The listing builds one solid part. Answer for the finished solid, in the listing's coordinates (mm). Coordinates: 2 decimals unless noted, no trailing zeros. Loops run counter-clockwise (first coordinate to the right, second up) from the corner with the lowest first, then second, coordinate; pieces in that order, holes last. Notation, with made-up numbers: M 42.25,55 L 99.25,55 A19 ccw 99.25,65 Z; hole C -18,-19.5 d1. An arc over 180 degrees is marked long. Return JSON: item names as keys, results as strings. Group by question number.
1. Section B-B (y = 124) is taken. Write down the section's boundary in (x, z).
2. Straight lines are drawn through the part: L1, parallel to Y at x = 82.5, z = 3.5; L2, parallel to X at y = 96, z = 3.8; L3, parallel to Y at x = 133, z = 1.1. For each, find the intervals that lie inside material, in ascending order. Write a range as from..to.
3. Section A-A (y = 19.05) is taken. Write down the section's boundary in (x, z) (3 decimals).
4. Given P1, Ø2, axis at x = 85.5, z = 1.5, coming from the +Y side; P2, Ø2, axis at x = 2, z = 2, coming from the +Y side; P3, Ø2, axis at y = 75.5, z = 1.5, coming from the +X side, each flat-ended and moving along its own axis, determine where each tip first touches the part or whether it passes through.
```python
from build123d import *

# Parameters (mm, degrees)
BOSS_EXTRUDE1_DEPTH = 4.4958
FILLET1_R           = 12.7
SKETCH2_W           = 4.4958
SKETCH2_H           = 12.7
CUT_EXTRUDE1_DEPTH  = 302.762747772
SKETCH3_W           = 12.7
SKETCH3_H           = 4.4958
CUT_EXTRUDE2_DEPTH  = 302.762747772
SKETCH4_R           = 5.08
CUT_EXTRUDE3_DEPTH  = 302.762747772
SKETCH5_W           = 25.4
SKETCH5_H           = 6.35
CUT_EXTRUDE4_DEPTH  = 302.762747772


with BuildPart() as part:
    # Sketch1 → Boss-Extrude1 (new body)
    with BuildSketch(Plane.XY):
        with BuildLine():
            Line((0, 114.3), (0, 0))
            Line((0, 0), (248.285, 0))
            Line((248.285, 0), (248.285, 114.3))
            ThreePointArc((248.285, 114.3), (207.873847455, 131.038847455), (191.135, 171.45))
            Line((191.135, 171.45), (57.15, 171.45))
            ThreePointArc((57.15, 171.45), (40.411152545, 131.038847455), (0, 114.3))
        make_face()
    extrude(amount=BOSS_EXTRUDE1_DEPTH)

    # Fillet1
    fillet1_edges = [part.edges().sort_by_distance(p)[0] for p in [
        (248.285, 114.3, 2.2479),
        (0, 114.3, 2.2479),
        (57.15, 171.45, 2.2479),
        (191.135, 171.45, 2.2479),
    ]]
    fillet(fillet1_edges, radius=FILLET1_R)

    # Sketch2 → Cut-Extrude1 (cut, through all)
    with BuildSketch(Plane.XY.offset(4.4958)):
        with Locations((246.0371, 96.414248202)):
            Rectangle(SKETCH2_W, SKETCH2_H)
        with Locations((246.0371, 77.364248202)):
            Rectangle(SKETCH2_W, SKETCH2_H)
        with Locations((246.0371, 39.264248202)):
            Rectangle(SKETCH2_W, SKETCH2_H)
        with Locations((246.0371, 58.314248202)):
            Rectangle(SKETCH2_W, SKETCH2_H)
        with Locations((246.0371, 20.214248202)):
            Rectangle(SKETCH2_W, SKETCH2_H)
        with Locations((2.2479, 96.414248202)):
            Rectangle(SKETCH2_W, SKETCH2_H)
        with Locations((2.2479, 77.364248202)):
            Rectangle(SKETCH2_W, SKETCH2_H)
        with Locations((2.2479, 58.314248202)):
            Rectangle(SKETCH2_W, SKETCH2_H)
        with Locations((2.2479, 39.264248202)):
            Rectangle(SKETCH2_W, SKETCH2_H)
        with Locations((2.2479, 20.214248202)):
            Rectangle(SKETCH2_W, SKETCH2_H)
    extrude(amount=-CUT_EXTRUDE1_DEPTH, mode=Mode.SUBTRACT)

    # Sketch3 → Cut-Extrude2 (cut, through all)
    with BuildSketch(Plane.XY.offset(4.4958)):
        with Locations((112.006917266, 169.2021)):
            Rectangle(SKETCH3_W, SKETCH3_H)
        with Locations((87.735751798, 169.2021)):
            Rectangle(SKETCH3_W, SKETCH3_H)
        with Locations((136.278082734, 169.2021)):
            Rectangle(SKETCH3_W, SKETCH3_H)
        with Locations((160.549248202, 169.2021)):
            Rectangle(SKETCH3_W, SKETCH3_H)
    extrude(amount=-CUT_EXTRUDE2_DEPTH, mode=Mode.SUBTRACT)

    # Sketch4 → Cut-Extrude3 (cut, through all)
    with BuildSketch(Plane.XY.offset(4.4958)):
        with Locations((210.185, 19.05)):
            Circle(SKETCH4_R)
    extrude(amount=-CUT_EXTRUDE3_DEPTH, mode=Mode.SUBTRACT)

    # Sketch5 → Cut-Extrude4 (cut, through all)
    with BuildSketch(Plane.XY.offset(4.4958)):
        with Locations((124.1425, 3.175)):
            Rectangle(SKETCH5_W, SKETCH5_H)
    extrude(amount=-CUT_EXTRUDE4_DEPTH, mode=Mode.SUBTRACT)


solid = part.part
```
Worked out:
{
 "1": {"outline": "M 31.85,0 L 216.43,0 L 216.43,4.5 L 31.85,4.5 Z"},
 "2": {"L1": "0..166.95", "L2": "4.5..243.79", "L3": "6.35..166.95"},
 "3": {"outline": "M 4.496,0 L 205.105,0 L 205.105,4.496 L 4.496,4.496 Z; M 215.265,0 L 243.789,0 L 243.789,4.496 L 215.265,4.496 Z"},
 "4": {"P1": "y = 166.95", "P2": "y = 110.96", "P3": "x = 243.79"}
}
